Design review of the part built by this model. Coordinates are the model's own, in mm. Face numbers are marked on the shaded views. A direction names the side the tool comes from. Coordinates: 2 decimals unless noted, no trailing zeros. Loops run counter-clockwise (first coordinate to the right, second up) from the corner with the lowest first, then second, coordinate; pieces in that order, holes last. Notation, with made-up numbers: (25.25, 33.25) - (58.25, 33.25) arc R24 ccw to (58.25, 58.25) - close; hole circle Ø3 at (75, 41.25). An arc over 180 degrees is marked (long way). One line per question, with ' | ' between items.
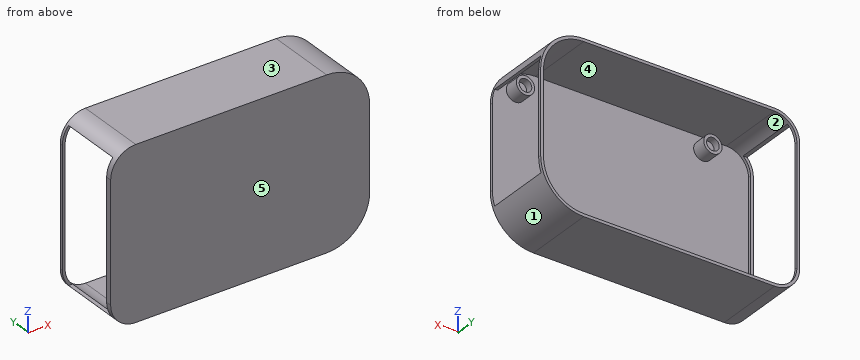
from build123d import *

# Parameters (mm, degrees)
BOSS_EXTRUDE1_DEPTH = 25
SKETCH1_3_R         = 2.225
BOSS_EXTRUDE2_DEPTH = 1
SKETCH1_4_R         = 3.225
BOSS_EXTRUDE3_DEPTH = 6
SKETCH2_R           = 2.225
CUT_EXTRUDE1_DEPTH  = 2.5
SKETCH3_W           = 39.21
SKETCH3_H           = 23
CUT_EXTRUDE2_DEPTH  = 4
SKETCH4_W           = 53.61
SKETCH4_H           = 22
CUT_EXTRUDE3_DEPTH  = 7


with BuildPart() as part:
    # Sketch1 → Boss-Extrude1 (new body)
    with BuildSketch(Plane(origin=(0, 0, 0), x_dir=(1, 0, 0), z_dir=(0, 1, 0))):
        with BuildLine():
            Line((-36.83, 29.805), (30.48, 29.805))
            ThreePointArc((30.48, 29.805), (41.228023074, 25.353023074), (45.68, 14.605))
            Line((45.68, 14.605), (45.68, -14.605))
            ThreePointArc((45.68, -14.605), (41.228023074, -25.353023074), (30.48, -29.805))
            Line((30.48, -29.805), (-36.83, -29.805))
            ThreePointArc((-36.83, -29.805), (-43.087895014, -27.212895014), (-45.68, -20.955))
            Line((-45.68, -20.955), (-45.68, 20.955))
            ThreePointArc((-45.68, 20.955), (-43.087895014, 27.212895014), (-36.83, 29.805))
        make_face()
        with BuildLine():
            Line((-36.83, 28.805), (30.48, 28.805))
            ThreePointArc((30.48, 28.805), (40.520916293, 24.645916293), (44.68, 14.605))
            Line((44.68, 14.605), (44.68, -14.605))
            ThreePointArc((44.68, -14.605), (40.520916293, -24.645916293), (30.48, -28.805))
            Line((30.48, -28.805), (-36.83, -28.805))
            ThreePointArc((-36.83, -28.805), (-42.380788232, -26.505788232), (-44.68, -20.955))
            Line((-44.68, -20.955), (-44.68, 20.955))
            ThreePointArc((-44.68, 20.955), (-42.380788232, 26.505788232), (-36.83, 28.805))
        make_face(mode=Mode.SUBTRACT)
    extrude(amount=BOSS_EXTRUDE1_DEPTH)

    # Sketch1_3 → Boss-Extrude2 (add)
    # profile 1 of 10: a face of its own
    with BuildSketch(Plane(origin=(0, 0, 0), x_dir=(1, 0, 0), z_dir=(0, 1, 0))):
        with BuildLine():
            ThreePointArc((30.48, 28.805), (40.520916293, 24.645916293), (44.68, 14.605))
            Line((44.68, 14.605), (44.68, -14.605))
            ThreePointArc((44.68, -14.605), (40.520916293, -24.645916293), (30.48, -28.805))
            Line((30.48, -28.805), (-36.83, -28.805))
            ThreePointArc((-36.83, -28.805), (-42.380788232, -26.505788232), (-44.68, -20.955))
            Line((-44.68, -20.955), (-44.68, 20.955))
            ThreePointArc((-44.68, 20.955), (-42.380788232, 26.505788232), (-36.83, 28.805))
            Line((-36.83, 28.805), (30.48, 28.805))
        make_face()
        with BuildLine():
            ThreePointArc((-36.83, 27.305), (-41.320128061, 25.445128061), (-43.18, 20.955))
            Line((-43.18, 20.955), (-43.18, -20.955))
            ThreePointArc((-43.18, -20.955), (-41.320128061, -25.445128061), (-36.83, -27.305))
            Line((-36.83, -27.305), (30.48, -27.305))
            ThreePointArc((30.48, -27.305), (39.460256121, -23.585256121), (43.18, -14.605))
            Line((43.18, -14.605), (43.18, 14.605))
            ThreePointArc((43.18, 14.605), (39.460256121, 23.585256121), (30.48, 27.305))
            Line((30.48, 27.305), (-36.83, 27.305))
        make_face(mode=Mode.SUBTRACT)
    # profile 2 of 10: a face of its own
    with BuildSketch(Plane(origin=(0, 0, 0), x_dir=(1, 0, 0), z_dir=(0, 1, 0))):
        with BuildLine():
            Line((-36.83, 27.305), (30.48, 27.305))
            ThreePointArc((30.48, 27.305), (39.460256121, 23.585256121), (43.18, 14.605))
            Line((43.18, 14.605), (43.18, -14.605))
            ThreePointArc((43.18, -14.605), (39.460256121, -23.585256121), (30.48, -27.305))
            Line((30.48, -27.305), (-36.83, -27.305))
            ThreePointArc((-36.83, -27.305), (-41.320128061, -25.445128061), (-43.18, -20.955))
            Line((-43.18, -20.955), (-43.18, 20.955))
            ThreePointArc((-43.18, 20.955), (-41.320128061, 25.445128061), (-36.83, 27.305))
        make_face()
        with Locations((-28.57, 24.265)):
            Circle(SKETCH1_3_R, mode=Mode.SUBTRACT)
        with Locations((37.53, 20.955)):
            Circle(SKETCH1_3_R, mode=Mode.SUBTRACT)
        with Locations((37.53, -20.955)):
            Circle(SKETCH1_3_R, mode=Mode.SUBTRACT)
        with Locations((-28.57, -24.125)):
            Circle(SKETCH1_3_R, mode=Mode.SUBTRACT)
    # profile 3 of 10: a face of its own
    with BuildSketch(Plane(origin=(0, 0, 0), x_dir=(1, 0, 0), z_dir=(0, 1, 0))):
        with BuildLine():
            Line((-27.493419766, 27.305), (-29.646580234, 27.305))
            ThreePointArc((-29.646580234, 27.305), (-30.431270231, 21.631314725), (-25.345, 24.265))
            ThreePointArc((-25.345, 24.265), (-25.936314725, 26.126270231), (-27.493419766, 27.305))
        make_face()
        with Locations((-28.57, 24.265)):
            Circle(SKETCH1_3_R, mode=Mode.SUBTRACT)
    # profile 4 of 10: a face of its own
    with BuildSketch(Plane(origin=(0, 0, 0), x_dir=(1, 0, 0), z_dir=(0, 1, 0))):
        with Locations((-28.57, 24.265)):
            Circle(SKETCH1_3_R)
    # profile 5 of 10: a face of its own
    with BuildSketch(Plane(origin=(0, 0, 0), x_dir=(1, 0, 0), z_dir=(0, 1, 0))):
        with BuildLine():
            ThreePointArc((-25.345, -24.125), (-30.651974118, -21.662073129), (-29.106865905, -27.305))
            Line((-29.106865905, -27.305), (-28.033134095, -27.305))
            ThreePointArc((-28.033134095, -27.305), (-26.107073129, -26.206974118), (-25.345, -24.125))
        make_face()
        with Locations((-28.57, -24.125)):
            Circle(SKETCH1_3_R, mode=Mode.SUBTRACT)
    # profile 6 of 10: a face of its own
    with BuildSketch(Plane(origin=(0, 0, 0), x_dir=(1, 0, 0), z_dir=(0, 1, 0))):
        with Locations((-28.57, -24.125)):
            Circle(SKETCH1_3_R)
    # profile 7 of 10: a face of its own
    with BuildSketch(Plane(origin=(0, 0, 0), x_dir=(1, 0, 0), z_dir=(0, 1, 0))):
        with BuildLine():
            ThreePointArc((40.755, -20.955), (34.583818023, -19.643269555), (39.687938443, -23.351649052))
            ThreePointArc((39.687938443, -23.351649052), (39.916507142, -23.104548986), (40.138446936, -22.851478205))
            ThreePointArc((40.138446936, -22.851478205), (40.596990901, -21.952091678), (40.755, -20.955))
        make_face()
        with Locations((37.53, -20.955)):
            Circle(SKETCH1_3_R, mode=Mode.SUBTRACT)
    # profile 8 of 10: a face of its own
    with BuildSketch(Plane(origin=(0, 0, 0), x_dir=(1, 0, 0), z_dir=(0, 1, 0))):
        with Locations((37.53, -20.955)):
            Circle(SKETCH1_3_R)
    # profile 9 of 10: a face of its own
    with BuildSketch(Plane(origin=(0, 0, 0), x_dir=(1, 0, 0), z_dir=(0, 1, 0))):
        with BuildLine():
            ThreePointArc((40.138446936, 22.851478205), (39.916507142, 23.104548986), (39.687938443, 23.351649052))
            ThreePointArc((39.687938443, 23.351649052), (34.583818023, 19.643269555), (40.755, 20.955))
            ThreePointArc((40.755, 20.955), (40.596990901, 21.952091678), (40.138446936, 22.851478205))
        make_face()
        with Locations((37.53, 20.955)):
            Circle(SKETCH1_3_R, mode=Mode.SUBTRACT)
    # profile 10 of 10: a face of its own
    with BuildSketch(Plane(origin=(0, 0, 0), x_dir=(1, 0, 0), z_dir=(0, 1, 0))):
        with Locations((37.53, 20.955)):
            Circle(SKETCH1_3_R)
    extrude(amount=BOSS_EXTRUDE2_DEPTH)

    # Sketch1_4 → Boss-Extrude3 (add)
    with BuildSketch(Plane(origin=(0, 0, 0), x_dir=(1, 0, 0), z_dir=(0, 1, 0))):
        with Locations(Location((-28.57, 24.265, 0), (0, 0, 270))):
            Circle(SKETCH1_4_R)
        with Locations(Location((-28.57, -24.125, 0), (0, 0, 270))):
            Circle(SKETCH1_4_R)
        with Locations(Location((37.53, -20.955, 0), (0, 0, 270))):
            Circle(SKETCH1_4_R)
        with Locations(Location((37.53, 20.955, 0), (0, 0, 270))):
            Circle(SKETCH1_4_R)
    extrude(amount=BOSS_EXTRUDE3_DEPTH)

    # Sketch2 → Cut-Extrude1 (cut)
    with BuildSketch(Plane(origin=(0, 6, 0), x_dir=(1, 0, 0), z_dir=(0, 1, 0))):
        with Locations(Location((-28.57, 24.265, 0), (0, 0, 270))):
            Circle(SKETCH2_R)
        with Locations(Location((-28.57, -24.125, 0), (0, 0, 270))):
            Circle(SKETCH2_R)
        with Locations(Location((37.53, -20.955, 0), (0, 0, 270))):
            Circle(SKETCH2_R)
        with Locations(Location((37.53, 20.955, 0), (0, 0, 270))):
            Circle(SKETCH2_R)
    extrude(amount=-CUT_EXTRUDE1_DEPTH, mode=Mode.SUBTRACT)

    # Sketch3 → Cut-Extrude2 (cut)
    with BuildSketch(Plane(origin=(45.68, 0, 0), x_dir=(0, 0, -1), z_dir=(1, 0, 0))):
        with Locations((0, 12.5)):
            Rectangle(SKETCH3_W, SKETCH3_H)
    extrude(amount=-CUT_EXTRUDE2_DEPTH, mode=Mode.SUBTRACT)

    # Sketch4 → Cut-Extrude3 (cut)
    with BuildSketch(Plane.ZY.offset(45.68)):
        with Locations((0, 13)):
            Rectangle(SKETCH4_W, SKETCH4_H)
    extrude(amount=-CUT_EXTRUDE3_DEPTH, mode=Mode.SUBTRACT)


solid = part.part
Q1. Tool access review of the marked faces 4 and 5: name each direction out of +Z, -Z, +X, -X, +Y, -Y from which nothing blocks a thin tool from reaching the whole face with its end or side.
Returned:
face 4: +Y | face 5: +Z, -Z, +X, -X, -Y
Q2. To check wall thickness, follow line 1 along Z through (x, y) = (25.5, 24) (3 decimals); line 2 along Y through (x, z) = (29, 5.5); line 3 along Z through (x, y) = (-38, 14.25). State the ranges of each line that lie inside material, in increasing order.
Returned:
line 1: z = -29.805 to -28.805, 28.805 to 29.805 | line 2: y = 0 to 1 | line 3: z = -29.73 to -28.72, 28.72 to 29.73
Q3. Take a section at C-C (x = 3). Give the boundary of the cut face in (y, z) (3 decimals), plus the area to 3 significant figures.
Returned:
outline: (0, -29.805) - (25, -29.805) - (25, -28.805) - (1, -28.805) - (1, 28.805) - (25, 28.805) - (25, 29.805) - (0, 29.805) - close | area: 108 mm²
Q4. Draft analysis for pull direction X (two halves, no side actions). For the marked faces 1, 2 and 3, state which applies: +X half, -X half, draft (parallel to the pull), parting line (faces both ways), or undercut.
Returned:
face 1: +X half | face 2: undercut | face 3: draft
Q5. For pin 1 (1 mm diameter, centred on y = 22, z = 24, fed in from -X); pin 2 (1.9 mm diameter, centred on x = -28, z = 23.5, fed in from +Y); pin 3 (12 mm diameter, centred on y = 21, z = 23, fed in from +X), all flat-tipped, find the tip position at first contact; note any pin that passes through.
Returned:
pin 1: stops at x = 40.66 | pin 2: stops at y = 3.5 | pin 3: stops at x = 45.34
Q6. Take a section at D-D (x = -28.57). Give the boundary of the cut face in (y, z) (3 decimals), plus the area to 3 significant figures.
Returned:
outline: (0, -29.805) - (25, -29.805) - (25, -28.805) - (1, -28.805) - (1, -27.49) - (6, -27.49) - (6, -26.49) - (3.5, -26.49) - (3.5, -22.04) - (6, -22.04) - (6, -21.04) - (1, -21.04) - (1, 20.9) - (6, 20.9) - (6, 21.9) - (3.5, 21.9) - (3.5, 26.35) - (6, 26.35) - (6, 27.35) - (1, 27.35) - (1, 28.805) - (25, 28.805) - (25, 29.805) - (0, 29.805) - close | area: 150 mm²
Q7. Take a section at B-B (z = -4.5). Give the boundary of the cut face in (x, y), plus the area to 3 significant figures.
Returned:
outline: (-45.68, 0) - (45.68, 0) - (45.68, 1) - (-44.68, 1) - (-44.68, 2) - (-45.68, 2) - close; (-45.68, 24) - (-44.68, 24) - (-44.68, 25) - (-45.68, 25) - close; (44.68, 24) - (45.68, 24) - (45.68, 25) - (44.68, 25) - close | area: 94.4 mm²
